Design review of the part built by this model. Coordinates are the model's own, in mm. Round coordinates to 2 decimals unless told otherwise and drop trailing zeros. Loops run counter-clockwise (first coordinate to the right, second up) from the corner with the lowest first, then second, coordinate; pieces in that order, holes last. Notation, with made-up numbers: (-25.5, -26) -> (7.5, -26) arc R13 cw to (7.5, -17) -> close; hole circle Ø8 at (-3, 38.25). An arc over 180 degrees is marked (long way). Use a Markdown table: item, result. Add a question column.
from build123d import *

# Parameters (mm, degrees)
F0_W     = 300
F0_H     = 150
F1_DEPTH = 70
F2_R     = 50
F3_R     = 5
F4_R     = 2


with BuildPart() as f1:
    # F0 (on Top) → F1 (new body)
    with BuildSketch(Plane.XY):
        with Locations((150, 78.7498958572)):
            Rectangle(F0_W, F0_H)
    extrude(amount=F1_DEPTH)

    # F2
    f2_edges = [f1.edges().sort_by_distance(p)[0] for p in [
        (0, 78.749896, 70),
        (300, 78.749896, 70),
    ]]
    fillet(f2_edges, radius=F2_R)

    # F3
    f3_edges = [f1.edges().sort_by_distance(p)[0] for p in [
        (0, 78.749896, 0),
        (300, 78.749896, 0),
    ]]
    fillet(f3_edges, radius=F3_R)

    # F4
    f4_edges = [f1.edges().sort_by_distance(p)[0] for p in [
        (150, 3.749896, 70),
        (150, 153.749896, 70),
        (150, 3.749896, 0),
        (150, 153.749896, 0),
        (300, 3.749896, 12.5),
        (300, 153.749896, 12.5),
        (0, 3.749896, 12.5),
        (1.464466, 3.749896, 1.464466),
        (14.644661, 3.749896, 55.355339),
        (298.535534, 3.749896, 1.464466),
        (285.355339, 3.749896, 55.355339),
        (298.535534, 153.749896, 1.464466),
        (285.355339, 153.749896, 55.355339),
        (1.464466, 153.749896, 1.464466),
        (14.644661, 153.749896, 55.355339),
        (0, 153.749896, 12.5),
    ]]
    fillet(f4_edges, radius=F4_R)


solid = f1.part
1. Consider section A-A on y = 130.5. State the section outline as (x, z) points.
2. To check wall thickness, follow probe 1 along X at (y, z) = (56, 22.5); probe 2 along Z at (x, y) = (264, 131.5); probe 3 along X at (y, z) = (50.5, 45.5). State the ranges of each line that lie inside material, in increasing order. Write a range as from..to.
3. Insertion check: P1, Ø1.5, axis at x = 265.5, y = 33.5, coming from the +Z side; P2, Ø1.5, axis at y = 122.5, z = 37.5, coming from the -X side. Each pin has a flat end and moves straight along its axis. Give the tip position at first contact, or say it passes through.
Verdict:
| question | item | result |
|---|---|---|
| 1 | outline | (0, 5) arc R5 ccw to (5, 0) -> (295, 0) arc R5 ccw to (300, 5) -> (300, 20) arc R50 ccw to (250, 70) -> (50, 70) arc R50 ccw to (0, 20) -> close |
| 2 | probe 1 | x = 0.06..299.94 |
| 2 | probe 2 | z = 0..68 |
| 2 | probe 3 | x = 6.99..293.01 |
| 3 | P1 | stops at z = 67.77 |
| 3 | P2 | stops at x = 2.89 |
